Design review of the part built by this model. Coordinates are the model's own, in mm. A direction names the side the tool comes from. Coordinates: 2 decimals unless noted, no trailing zeros. Order: outer loops, then holes, each group sorted by start corner. A loop starts at its lowest first (then second) coordinate and runs counter-clockwise, first axis right, second up. Notation, with made-up numbers: (41, -10) -> (93, -10) arc R11 ccw to (93, -5) -> close; hole circle Ø5 at (61.5, 49.25). An arc over 180 degrees is marked (long way). Write item = value, one per line.
```python
from build123d import *

# Parameters (mm, degrees)
SKETCH1_W           = 40
SKETCH1_H           = 20
BOSS_EXTRUDE1_DEPTH = 40
CUT_EXTRUDE1_DEPTH  = 40
CUT_EXTRUDE2_DEPTH  = 40
BOSS_EXTRUDE2_DEPTH = 20
BOSS_EXTRUDE3_DEPTH = 20
SKETCH6_W           = 40
SKETCH6_H           = 40
CUT_EXTRUDE3_DEPTH  = 20
SKETCH7_W           = 28.284271247
SKETCH7_H           = 20
CUT_EXTRUDE4_DEPTH  = 20
SKETCH8_W           = 20
SKETCH8_H           = 20
CUT_EXTRUDE5_DEPTH  = 20
CUT_EXTRUDE6_DEPTH  = 20
CUT_EXTRUDE7_DEPTH  = 20
SKETCH11_W          = 20
SKETCH11_H          = 20
CUT_EXTRUDE8_DEPTH  = 20
SKETCH12_W          = 20
SKETCH12_H          = 20
BOSS_EXTRUDE4_DEPTH = 20
CUT_EXTRUDE9_DEPTH  = 20
CUT_EXTRUDE10_DEPTH = 20


with BuildPart() as part:
    # Sketch1 → Boss-Extrude1 (new body)
    with BuildSketch(Plane.XY):
        with Locations((20, 10)):
            Rectangle(SKETCH1_W, SKETCH1_H)
    extrude(amount=BOSS_EXTRUDE1_DEPTH)

    # Sketch2 → Cut-Extrude1 (cut)
    with BuildSketch(Plane(origin=(0, 20, 0), x_dir=(1, 0, 0), z_dir=(0, 1, 0))):
        Polygon((0, -20), (20, -40), (0, -40), align=None)
    extrude(amount=-CUT_EXTRUDE1_DEPTH, mode=Mode.SUBTRACT)

    # Sketch3 → Cut-Extrude2 (cut)
    with BuildSketch(Plane(origin=(0, 20, 0), x_dir=(1, 0, 0), z_dir=(0, 1, 0))):
        Polygon((20, -40), (20, -20), (0, -20), align=None)
    extrude(amount=-CUT_EXTRUDE2_DEPTH, mode=Mode.SUBTRACT)

    # Sketch4 → Boss-Extrude2 (add)
    with BuildSketch(Plane(origin=(0, 20, 0), x_dir=(1, 0, 0), z_dir=(0, 1, 0))):
        Polygon((0, 0), (0, -20), (40, -20), (20, 0), align=None)
    extrude(amount=BOSS_EXTRUDE2_DEPTH)

    # Sketch5 → Boss-Extrude3 (add)
    with BuildSketch(Plane(origin=(-8.888888889, 4.444444444, 8.888888889), x_dir=(0.745355992, 0.298142397, 0.596284794), z_dir=(-0.666666667, 0.333333333, 0.666666667))):
        Polygon((11.92569588, -8.94427191), (38.75851161, -17.88854382), (38.75851161, 26.83281573), align=None)
    extrude(amount=-BOSS_EXTRUDE3_DEPTH)

    # Sketch6 → Cut-Extrude3 (cut)
    with BuildSketch(Plane.XZ):
        with Locations((20, 20)):
            Rectangle(SKETCH6_W, SKETCH6_H)
    extrude(amount=CUT_EXTRUDE3_DEPTH, mode=Mode.SUBTRACT)

    # Sketch7 → Cut-Extrude4 (cut)
    with BuildSketch(Plane(origin=(10, 0, -10), x_dir=(-0.707106781, 0, -0.707106781), z_dir=(0.707106781, 0, -0.707106781))):
        with Locations((-28.284271248, 30)):
            Rectangle(SKETCH7_W, SKETCH7_H)
    extrude(amount=CUT_EXTRUDE4_DEPTH, mode=Mode.SUBTRACT)

    # Sketch8 → Cut-Extrude5 (cut)
    with BuildSketch(Plane(origin=(20, 0, 0), x_dir=(0, 0, -1), z_dir=(1, 0, 0))):
        with Locations((-30, 30)):
            Rectangle(SKETCH8_W, SKETCH8_H)
    extrude(amount=CUT_EXTRUDE5_DEPTH, mode=Mode.SUBTRACT)

    # Sketch9 → Cut-Extrude6 (cut)
    with BuildSketch(Plane.XY.offset(20)):
        Polygon((0, 40), (0, 20), (10, 20), (20, 40), align=None)
    extrude(amount=-CUT_EXTRUDE6_DEPTH, mode=Mode.SUBTRACT)

    # Sketch10 → Cut-Extrude7 (cut)
    with BuildSketch(Plane(origin=(0, 20, 0), x_dir=(1, 0, 0), z_dir=(0, 1, 0))):
        Polygon((40, 0), (40, -20), (20, 0), align=None)
    extrude(amount=-CUT_EXTRUDE7_DEPTH, mode=Mode.SUBTRACT)

    # Sketch11 → Cut-Extrude8 (cut)
    with BuildSketch(Plane.XY.offset(20)):
        with Locations((30, 30)):
            Rectangle(SKETCH11_W, SKETCH11_H)
    extrude(amount=-CUT_EXTRUDE8_DEPTH, mode=Mode.SUBTRACT)

    # Sketch12 → Boss-Extrude4 (add)
    with BuildSketch(Plane.XY.offset(40)):
        with Locations((30, 30)):
            Rectangle(SKETCH12_W, SKETCH12_H)
    extrude(amount=-BOSS_EXTRUDE4_DEPTH)

    # Sketch14 → Cut-Extrude9 (cut)
    with BuildSketch(Plane(origin=(20, 0, 0), x_dir=(0, 0, -1), z_dir=(1, 0, 0))):
        Polygon((-20, 40), (-10, 30), (0, 40), align=None)
        Polygon((0, 40), (-10, 30), (0, 20), align=None)
    extrude(amount=-CUT_EXTRUDE9_DEPTH, mode=Mode.SUBTRACT)

    # Sketch15 → Cut-Extrude10 (cut)
    with BuildSketch(Plane.ZY.offset(-20)):
        Polygon((20, 40), (40, 0), (40, 40), align=None)
    extrude(amount=-CUT_EXTRUDE10_DEPTH, mode=Mode.SUBTRACT)


solid = part.part
```
(1) We need section D-D (y = 27). Write out the cut boundary in (x, z).
Report:
outline = (13.5, 7) -> (20, 7) -> (20, 20) -> (40, 20) -> (40, 26.5) -> (20, 26.5) -> (13.5, 20) -> close
(2) We need section A-A (y = 4). Write out the cut boundary in (x, z), and give its area (3 significant figures).
Report:
outline = (0, 0) -> (20, 0) -> (40, 20) -> (40, 38) -> (20, 38) -> (2, 20) -> (0, 20) -> close
area = 1,120 mm²
(3) We need section C-C (x = 17.5). Write out the cut boundary in (y, z).
Report:
outline = (0, 0) -> (20, 0) -> (35, 15) -> (35, 20) -> (0, 37.5) -> close
(4) Insertion check: pin 1 (6 mm diameter, centred on x = 35, y = 11.5, fed in from -Z); pin 2 (3 mm diameter, centred on x = 14.5, y = 17, fed in from +Z); pin 3 (11 mm diameter, centred on x = 7, z = 7, fed in from +Y). Each pin has a flat end and moves straight along its axis. Give the tip position at first contact, or say it passes through.
Report:
pin_1 = 12
pin_2 = 27.68
pin_3 = 25
(5) For L1, parallel to Y at x = 25.5, z = 13; L2, parallel to X at y = 15, z = 7; L3, parallel to Y at x = 26.5, z = 37.5, list the stretches that pass through material, from the lowest coordinate up.
Report:
L1 = 0 to 20
L2 = 0 to 27
L3 = 0 to 5
(6) We need section B-B (z = 14.5). Write out the cut boundary in (x, y).
Report:
outline = (0, 0) -> (34.5, 0) -> (34.5, 20) -> (20, 20) -> (20, 34.5) -> (17.25, 34.5) -> (10, 20) -> (0, 20) -> close
(7) For faces 1 (the flat face through (5, 20, 10)), 2 (the flat face through (25, 20, 14)), 3 (the flat face through (3, 14, 20)), list the 3-axis set-ups (+Z, -Z, +X, -X, +Y, -Y) from which the entire face can be reached by the end or side of a thin tool; tool diameter is ignored.
Report:
face_1 = +Z, -Z, -X, +Y
face_2 = -Z, +X, +Y
face_3 = +Z, -X, +Y
